Input: dimensioned drawing with shaded views. Units: mm. Origin: part minimum x, y, z. A direction names the side the tool comes from. Coordinates: 2 decimals unless noted, no trailing zeros. Write each loop counter-clockwise with the first axis right and the second up, starting at its lowest first coordinate (ties: lowest second). Pieces come first, ordered by that corner, then holes. Notation, with made-up numbers: M 23.25,26.5 L 56.25,26.5 A20 ccw 56.25,43.5 Z; hole C -2.5,76.25 d2. An arc over 180 degrees is marked long. Write each question's results on one line, items separated by ' | '. Start each with the question number.
1. Section query A-A, the plane y = 2.8. Output: boundary loops of the cut face in (x, z), and give its area (3 significant figures).
2. Section query B-B, the plane x = 2.8. Output: boundary loops of the cut face in (y, z), and give its area (3 significant figures).
3. Set-up query: the marked faces 4, 5 and 6. Return all of +Z, -Z, +X, -X, +Y, -Y with unobstructed straight access to the full face (end or side cutting, diameter ignored); none if empty.
4. Pull-direction query (Y, two-part tool) for the marked faces 1, 2 and 3; classes: +Y half, -Y half, draft (parallel to the pull), parting line (faces both ways), or undercut.
5. Ray query, probe 1 along Y at (x, z) = (2.8, 0.3); probe 2 along Z at (x, y) = (2.65, 4); probe 3 along Z at (x, y) = (3.1, 5.75). Return the intervals inside material, ascending.
6. Section query C-C, the plane z = 1.85. Output: boundary loops of the cut face in (x, y).
7. First-contact query: pin 1 (0.8 mm diameter, centred on x = 3, y = 2.5, fed in from -Z); pin 2 (1 mm diameter, centred on x = 4, y = 5.5, fed in from -Z); pin 3 (1 mm diameter, centred on y = 1.5, z = 1.5, fed in from +X). Flat tips, straight axial feed; report the tip coordinate or a pass-through.
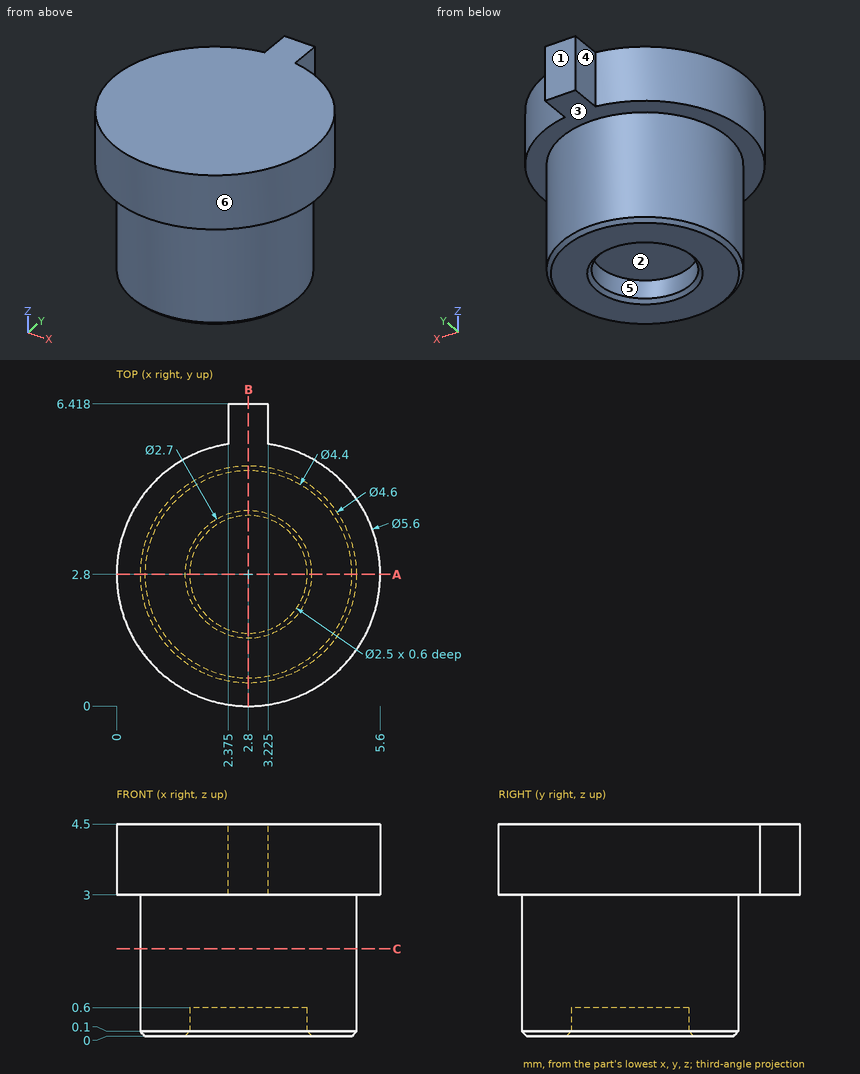
Answer:
1) outline: M 0,3 L 0.5,3 L 0.5,0.1 L 0.6,0 L 1.45,0 L 1.55,0.1 L 1.55,0.6 L 4.05,0.6 L 4.05,0.1 L 4.15,0 L 5,0 L 5.1,0.1 L 5.1,3 L 5.6,3 L 5.6,4.5 L 0,4.5 Z | area: 20.7 mm^2
2) outline: M 0,3 L 0.5,3 L 0.5,0.1 L 0.6,0 L 1.45,0 L 1.55,0.1 L 1.55,0.6 L 4.05,0.6 L 4.05,0.1 L 4.15,0 L 5,0 L 5.1,0.1 L 5.1,3 L 6.42,3 L 6.42,4.5 L 0,4.5 Z | area: 21.9 mm^2
3) face 4: +Z, -Z, -X, +Y | face 5: -Z | face 6: +Z, -Z
4) face 1: +Y half | face 2: undercut | face 3: draft
5) probe 1: 0.5 to 1.55, 4.05 to 5.1 | probe 2: 0.6 to 4.5 | probe 3: 3 to 4.5
6) outline: C 2.8,2.8 d4.6
7) pin 1: z = 0.6 | pin 2: z = 3 | pin 3: x = 4.96
